Can you work these out from the drawing? Everything is in mm from the part's minimum corner. Round coordinates to 2 decimals unless told otherwise and drop trailing zeros. Write each loop counter-clockwise with the first axis right and the second up, starting at its lowest first coordinate (ties: lowest second). Pieces come first, ordered by that corner, then holes. Notation, with made-up numbers: (-3.75, -32.75) -> (11.25, -32.75) arc R21 ccw to (11.25, 3.25) -> close; hole circle Ø8 at (70.25, 17.5). An arc over 180 degrees is marked (long way). Put each result on its own line as item: value. Start each with the question number.
1. Suppose I cut it at C-C (y = 14). Please give me the cut outline in (x, z), then the cut area to 3 significant figures.
2. I need wall thicknesses on probe 1 along X at (y, z) = (11, 7.5); probe 2 along X at (y, z) = (9.5, 8.25); probe 3 along Z at (x, y) = (5.5, 8.5). Which ranges of each line are inside material? Lowest first, please. Write a range as from..to.
3. For pin 1 (0.5 mm diameter, centred on x = 14.5, y = 10, fed in from +Z); pin 2 (8 mm diameter, centred on y = 20, z = 2.5, fed in from +X); pin 3 (1.1 mm diameter, centred on x = 14.5, y = 13.5, fed in from -Z); pin 4 (1 mm diameter, centred on x = 8, z = 6, fed in from -Y), each with a flat end and sliding along its axis, tell me the tip position at first contact or that it passes through.
4. Suppose I cut it at A-A (z = 4.25). Please give me the cut outline in (x, y), then the cut area to 3 significant figures.
5. Suppose I cut it at B-B (x = 14.25). Please give me the cut outline in (y, z), then the cut area to 3 significant figures.
6. We'd pull the mould along Z, two halves only. Please class the marked faces 1, 2 and 3: +Z half, -Z half, draft (parallel to the pull), parting line (faces both ways), or undercut.
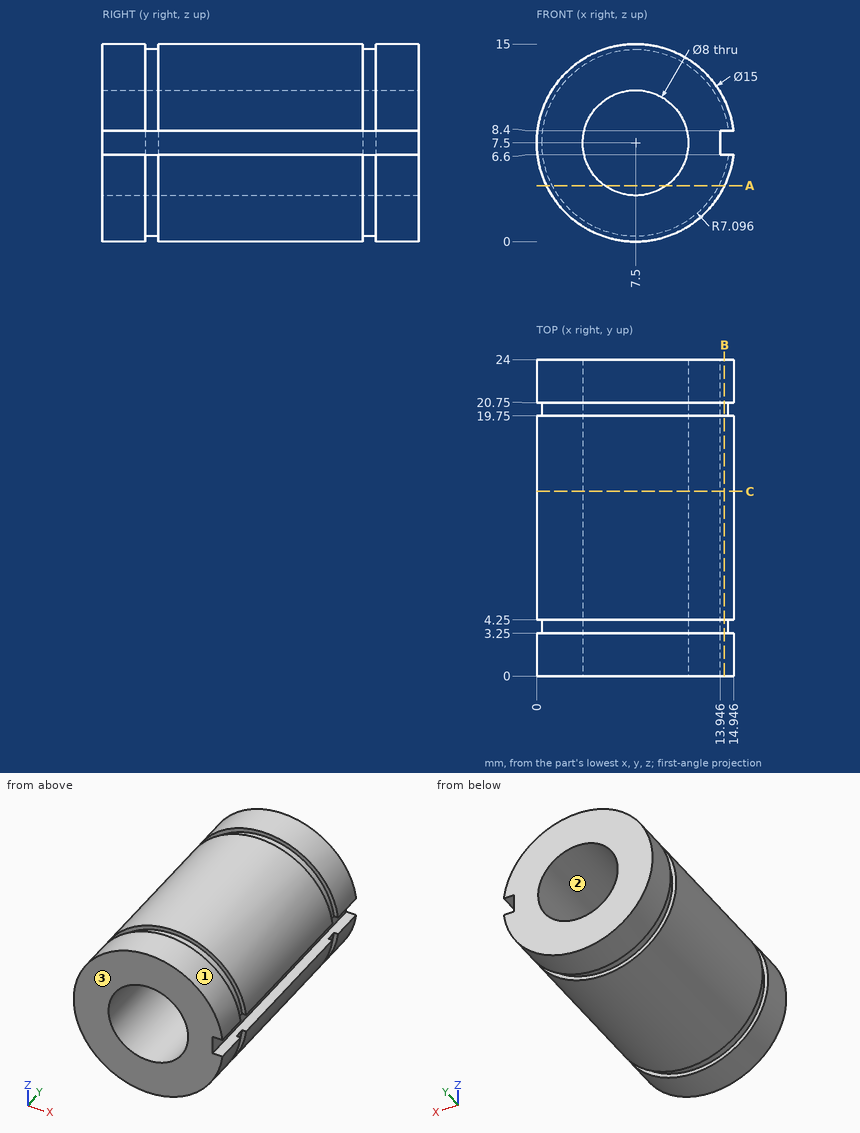
Verdict:
1. outline: (13.95, 6.6) -> (13.95, 8.4) -> (14.95, 8.4) arc R7.5 ccw (long way) to (14.95, 6.6) -> close; hole circle Ø8 at (7.5, 7.5)
1. area: 125 mm^2
2. probe 1: x = 0..3.5, 11.5..13.95
2. probe 2: x = 0.04..3.57, 11.43..13.95
2. probe 3: z = 0.27..4.04, 10.96..14.73
3. pin 1: stops at z = 10.77
3. pin 2: stops at x = 14.93
3. pin 3: stops at z = 3.67
3. pin 4: passes through
4. outline: (0.74, 0) -> (5.17, 0) -> (5.17, 24) -> (0.74, 24) -> (0.74, 20.75) -> (1.19, 20.75) -> (1.19, 19.75) -> (0.74, 19.75) -> (0.74, 4.25) -> (1.19, 4.25) -> (1.19, 3.25) -> (0.74, 3.25) -> close; (9.83, 0) -> (14.26, 0) -> (14.26, 3.25) -> (13.81, 3.25) -> (13.81, 4.25) -> (14.26, 4.25) -> (14.26, 19.75) -> (13.81, 19.75) -> (13.81, 20.75) -> (14.26, 20.75) -> (14.26, 24) -> (9.83, 24) -> close
4. area: 211 mm^2
5. outline: (0, 4.23) -> (3.25, 4.23) -> (3.25, 5.31) -> (4.25, 5.31) -> (4.25, 4.23) -> (19.75, 4.23) -> (19.75, 5.31) -> (20.75, 5.31) -> (20.75, 4.23) -> (24, 4.23) -> (24, 6.6) -> (0, 6.6) -> close; (0, 8.4) -> (24, 8.4) -> (24, 10.77) -> (20.75, 10.77) -> (20.75, 9.69) -> (19.75, 9.69) -> (19.75, 10.77) -> (4.25, 10.77) -> (4.25, 9.69) -> (3.25, 9.69) -> (3.25, 10.77) -> (0, 10.77) -> close
5. area: 109 mm^2
6. face 1: parting line
6. face 2: undercut
6. face 3: draft
